```python
from build123d import *

# Parameters (mm, degrees)
SKETCH1_R           = 1.8288
SKETCH1_R_2         = 4
SKETCH1_R_3         = 3
BOSS_EXTRUDE1_DEPTH = 3.175
CUT_EXTRUDE1_REACH  = 146.039
SKETCH2_W           = 4.112404804
SKETCH2_H           = 133.245584328
FILLET3_R           = 2.5
FILLET4_R           = 5


with BuildPart() as part:
    # Sketch1 → Boss-Extrude1 (new body)
    with BuildSketch(Plane(origin=(0, 0, 0), x_dir=(0, 0, -1), z_dir=(1, 0, 0))):
        with BuildLine():
            Line((20.757404804, -103.81), (20.757404804, -5))
            Line((20.757404804, -5), (7.5, 29.435584328))
            Line((7.5, 29.435584328), (7.5, 135))
            ThreePointArc((7.5, 135), (0, 142.5), (-7.5, 135))
            Line((-7.5, 135), (-7.5, 29.435584328))
            Line((-7.5, 29.435584328), (-20.757404804, -5))
            Line((-20.757404804, -5), (-20.757404804, -103.81))
            Line((-20.757404804, -103.81), (20.757404804, -103.81))
        make_face()
        with Locations((-13.4747, -100)):
            Circle(SKETCH1_R, mode=Mode.SUBTRACT)
        with Locations((13.4747, -100)):
            Circle(SKETCH1_R, mode=Mode.SUBTRACT)
        with Locations((13.4747, 0)):
            Circle(SKETCH1_R, mode=Mode.SUBTRACT)
        with Locations((-13.4747, 0)):
            Circle(SKETCH1_R, mode=Mode.SUBTRACT)
        with Locations((0, 35)):
            Circle(SKETCH1_R_2, mode=Mode.SUBTRACT)
        with Locations((0, 135)):
            Circle(SKETCH1_R_3, mode=Mode.SUBTRACT)
    extrude(amount=BOSS_EXTRUDE1_DEPTH)

    # Sketch2 → Cut-Extrude1 (cut, up to next)
    with BuildSketch(Plane(origin=(3.175, 0, 0), x_dir=(0, 0, -1), z_dir=(1, 0, 0)), mode=Mode.PRIVATE) as cut_extrude1_sk1:
        Polygon((11.645, -2.5), (-11.645, -2.5), (11.645, -26.921755536), align=None)
    cut_extrude1_tool1 = extrude(cut_extrude1_sk1.sketch, amount=-CUT_EXTRUDE1_REACH, mode=Mode.PRIVATE) & part.part
    # Sketch2 → Cut-Extrude1 (cut, up to next)
    with BuildSketch(Plane(origin=(3.175, 0, 0), x_dir=(0, 0, -1), z_dir=(1, 0, 0)), mode=Mode.PRIVATE) as cut_extrude1_sk2:
        Polygon((-11.645, -9.744911131), (11.645, -34.166666667), (-11.645, -58.588422203), (-11.645, -34.166666667), align=None)
    cut_extrude1_tool2 = extrude(cut_extrude1_sk2.sketch, amount=-CUT_EXTRUDE1_REACH, mode=Mode.PRIVATE) & part.part
    # Sketch2 → Cut-Extrude1 (cut, up to next)
    with BuildSketch(Plane(origin=(3.175, 0, 0), x_dir=(0, 0, -1), z_dir=(1, 0, 0)), mode=Mode.PRIVATE) as cut_extrude1_sk3:
        Polygon((-11.645, -73.078244464), (-11.645, -97.5), (11.645, -97.5), align=None)
    cut_extrude1_tool3 = extrude(cut_extrude1_sk3.sketch, amount=-CUT_EXTRUDE1_REACH, mode=Mode.PRIVATE) & part.part
    # Sketch2 → Cut-Extrude1 (cut, up to next)
    with BuildSketch(Plane(origin=(3.175, 0, 0), x_dir=(0, 0, -1), z_dir=(1, 0, 0)), mode=Mode.PRIVATE) as cut_extrude1_sk4:
        Polygon((11.645, -41.411577797), (11.645, -65.833333333), (11.645, -90.255088869), (-11.645, -65.833333333), align=None)
    cut_extrude1_tool4 = extrude(cut_extrude1_sk4.sketch, amount=-CUT_EXTRUDE1_REACH, mode=Mode.PRIVATE) & part.part
    # Sketch2 → Cut-Extrude1 (cut, up to next)
    with BuildSketch(Plane(origin=(3.175, 0, 0), x_dir=(0, 0, -1), z_dir=(1, 0, 0)), mode=Mode.PRIVATE) as cut_extrude1_sk5:
        with Locations((-18.701202402, -37.187207836)):
            Rectangle(SKETCH2_W, SKETCH2_H)
    cut_extrude1_tool5 = extrude(cut_extrude1_sk5.sketch, amount=-CUT_EXTRUDE1_REACH, mode=Mode.PRIVATE) & part.part
    # Sketch2 → Cut-Extrude1 (cut, up to next)
    with BuildSketch(Plane(origin=(3.175, 0, 0), x_dir=(0, 0, -1), z_dir=(1, 0, 0)), mode=Mode.PRIVATE) as cut_extrude1_sk6:
        with Locations((18.701202402, -37.187207836)):
            Rectangle(SKETCH2_W, SKETCH2_H)
    cut_extrude1_tool6 = extrude(cut_extrude1_sk6.sketch, amount=-CUT_EXTRUDE1_REACH, mode=Mode.PRIVATE) & part.part
    add(cut_extrude1_tool1.solids().sort_by_distance((3.175, -10.640585, -3.881667))[0], mode=Mode.SUBTRACT)
    add(cut_extrude1_tool2.solids().sort_by_distance((3.175, -34.166667, 3.881667))[0], mode=Mode.SUBTRACT)
    add(cut_extrude1_tool3.solids().sort_by_distance((3.175, -89.359415, 3.881667))[0], mode=Mode.SUBTRACT)
    add(cut_extrude1_tool4.solids().sort_by_distance((3.175, -65.833333, -3.881667))[0], mode=Mode.SUBTRACT)
    add(cut_extrude1_tool5.solids().sort_by_distance((3.175, -37.187208, 18.701202))[0], mode=Mode.SUBTRACT)
    add(cut_extrude1_tool6.solids().sort_by_distance((3.175, -37.187208, -18.701202))[0], mode=Mode.SUBTRACT)

    # Fillet3
    fillet3_edges = [part.edges().sort_by_distance(p)[0] for p in [
        (1.5875, -26.921755536, -11.645),
        (1.5875, -2.5, 11.645),
        (1.5875, -2.5, -11.645),
        (1.5875, -103.81, 16.645),
        (1.5875, -9.744911131, 11.645),
        (1.5875, -34.166666667, -11.645),
        (1.5875, -58.588422203, 11.645),
        (1.5875, -103.81, -16.645),
        (1.5875, -73.078244464, 11.645),
        (1.5875, -97.5, -11.645),
        (1.5875, -97.5, 11.645),
        (1.5875, -90.255088869, -11.645),
        (1.5875, -65.833333333, 11.645),
        (1.5875, -41.411577797, -11.645),
    ]]
    fillet(fillet3_edges, radius=FILLET3_R)

    # Fillet4
    fillet4_edges = [part.edges().sort_by_distance(p)[0] for p in [
        (1.5875, 29.435584328, -7.5),
        (1.5875, 29.435584328, 7.5),
        (1.5875, 5.681808734, 16.645),
        (1.5875, 5.681808734, -16.645),
    ]]
    fillet(fillet4_edges, radius=FILLET4_R)


solid = part.part
```
Geometry: final body of the model. Coordinates: model frame, mm. A direction names the side the tool comes from. Round coordinates to 2 decimals unless told otherwise and drop trailing zeros. Order: outer loops, then holes, each group sorted by start corner. A loop starts at its lowest first (then second) coordinate and runs counter-clockwise, first axis right, second up. Notation, with made-up numbers: M 73.5,16 L 121.5,16 A19 ccw 121.5,28 Z; hole C -1.75,75.5 d1. An arc over 180 degrees is marked long. One line per item, written item: value.
(1) Pin query (flat end, axial travel): P1, Ø3, axis at y = 0, z = 13.47, coming from the -X side; P2, Ø1.6, axis at x = 1, y = 64, coming from the +Z side. Return the tip coordinate at first contact, or that it passes through.
Result sheet:
P1: through
P2: z = 7.5
(2) Cut plane D-D (y = 112.5). Return the cut outline in (x, z) (3 decimals).
Result sheet:
outline: M 0,-7.5 L 3.175,-7.5 L 3.175,7.5 L 0,7.5 Z
(3) Reachability of faces 1 (the flat face through (1.61, -44.854, -1.453)), 2 (the cylindrical face through (1.57, 142.5, -0.16)) from +Z, -Z, +X, -X, +Y, -Y: full face, straight path, thin tool, end or side. Return the list, or none.
Result sheet:
face 1: +X, -X
face 2: +X, -X, +Y
(4) Pull-direction query (Y, two-part tool) for faces 3 (the flat face through (1.6, -85.5, -0.2)), 4 (the flat face through (1.565, 17.713, 12.013)), 5 (the flat face through (0, 21, 0)); classes: pulls with the +Y half, pulls with the -Y half, needs draft (parallel to the pull), parting line crosses it, or undercut.
Result sheet:
face 3: undercut
face 4: pulls with the +Y half
face 5: needs draft
(5) Cut plane B-B (z = 0). Return the cut outline in (x, y) (3 decimals), and give its area (3 significant figures).
Result sheet:
outline: M 0,-103.81 L 3.175,-103.81 L 3.175,-97.5 L 0,-97.5 Z; M 0,-85.289 L 3.175,-85.289 L 3.175,-78.044 L 0,-78.044 Z; M 0,-53.622 L 3.175,-53.622 L 3.175,-46.378 L 0,-46.378 Z; M 0,-21.956 L 3.175,-21.956 L 3.175,-14.711 L 0,-14.711 Z; M 0,-2.5 L 3.175,-2.5 L 3.175,31 L 0,31 Z; M 0,39 L 3.175,39 L 3.175,132 L 0,132 Z; M 0,138 L 3.175,138 L 3.175,142.5 L 0,142.5 Z
area: 505 mm2
(6) Cut plane A-A (y = 35). Return the cut outline in (x, z) (3 decimals), and give its area (3 significant figures).
Result sheet:
outline: M 0,-7.5 L 3.175,-7.5 L 3.175,-4 L 0,-4 Z; M 0,4 L 3.175,4 L 3.175,7.5 L 0,7.5 Z
area: 22.2 mm2
(7) Cut plane C-C (x = 2.5). Give the number of separate pieces and of enclosed holes in the cut face, and give its area (3 significant figures).
Result sheet:
separate pieces: 1
enclosed holes: 10
area: 4,130 mm2
(8) Line query: probe 1 along Z at (x, y) = (1.2, -100) (1 decimal); probe 2 along Z at (x, y) = (2.25, -82) (3 decimals); probe 3 along Y at (x, z) = (1.2, 5.5). Output: solid intervals per line, ascending. Write a range as [from, to].
Result sheet:
probe 1: [-16.6, -15.3], [-11.6, 11.6], [15.3, 16.6]
probe 2: [-16.645, -11.645], [-3.772, 3.137], [11.645, 16.645]
probe 3: [-103.81, -97.5], [-79.52, -72.28], [-59.39, -52.14], [-16.19, -8.94], [-2.5, 140.1]
